from build123d import *

# Parameters (mm, degrees)
SCREW_HOLES_COUNT = 12


with BuildPart() as part:
    # Cross Section → Main (revolve)
    with BuildSketch(Plane.XY):
        Polygon((-38.1, 0), (-38.1, -3.175), (-41.275, -3.175), (-41.275, -15.875), (-41.656, -15.215088642), (-41.656, -3.175), (-48.514, -3.175), (-48.514, 9.525), (-47.625, 9.525), (-47.625, 0), align=None)
    revolve(axis=Axis((0, 55, 0), (0, -1, 0)))

    # Sketch7 → #3-48 Tapped Hole1 (revolve, cut)
    with BuildSketch(Plane(origin=(-42.8625, 0, 0), x_dir=(0, 0, 1), z_dir=(1, 0, 0))):
        Polygon((0, 0), (0, 3.901027994), (0.99695, 3.302), (0.99695, 0), align=None)
    f_3_48_tapped_hole1 = revolve(axis=Axis((-42.8625, 6.35, 0), (0, -1, 0)), mode=Mode.SUBTRACT)

    # Screw Holes: #3-48 Tapped Hole1 ×12 about axis
    screw_holes_axis = Axis((0, 0, 0), (0, 1, 0))
    for i in range(1, SCREW_HOLES_COUNT):
        add(f_3_48_tapped_hole1.rotate(screw_holes_axis, i * 360 / SCREW_HOLES_COUNT), mode=Mode.SUBTRACT)


solid = part.part
Source: CAD feature listing. Evaluate the final solid. Frame: model axes, mm. A direction names the side the tool comes from. Give positions to 0.01 mm unless a question says otherwise; leave off trailing zeros. Write each loop counter-clockwise with the first axis right and the second up, starting at its lowest first coordinate (ties: lowest second). Pieces come first, ordered by that corner, then holes. Notation, with made-up numbers: (49, 61) - (62, 61) arc R21 ccw to (62, 81) - close; hole circle Ø2 at (84.25, 6.25). An arc over 180 degrees is marked (long way). Write item = value, one per line. Start each with the question number.
Q1. Draft query along Z for faces 1 (the cylindrical face through (-46.274, 3.264, -14.572)), 2 (the cylindrical face through (30.235, -1.61, 23.183)), 3 (the flat face through (14, -3.175, -40)). Return one class per face: +Z half, -Z half, draft (parallel to the pull), parting line (faces both ways), or undercut.
Q2. Cut plane A-A, the plane y = -1.25. Give the number of separate pieces and of enclosed holes in the cut face, then the cut area to 3 significant figures.
Q3. Pin query (flat end, axial travel): pin 1 Ø2 at (x, y) = (23, -11) entering from -Z; pin 2 Ø1 at (y, z) = (6.5, -20.5) entering from -X; pin 3 Ø2.5 at (x, z) = (-37.12, 21.43) entering from +Y. Return the tip coordinate at first contact, or that it passes through.
Q4. Reachability of faces 4 (the flat face through (14, 0, -36)), 5 (the flat face through (-36, 9.525, 32)), 6 (the cylindrical face through (-39.732, -9.111, -12.512)) from +Z, -Z, +X, -X, +Y, -Y: full face, straight path, thin tool, end or side. Return the list, or none.
Q5. Material intervals for probe 1 along Z at (x, y) = (0, -1.7); probe 2 along X at (y, z) = (-2.75, -43); probe 3 along X at (y, z) = (-11.25, 1), sorted ascending.
Q6. Cut plane B-B, the plane y = -9.25. Return loops of the section in (x, z) (3 decimals).
Computed values:
q1.face_1 = parting line
q1.face_2 = undercut
q1.face_3 = draft
q2.separate_pieces = 1
q2.enclosed_holes = 13
q2.area = 2,800 mm²
q3.pin_1 = -35.37
q3.pin_2 = -44.2
q3.pin_3 = 0
q4.face_4 = +Y
q4.face_5 = +Z, -Z, +X, -X, +Y
q4.face_6 = -Y
q5.probe_1 = -48.51 to -43.86, -41.87 to -38.1, 38.1 to 41.87, 43.86 to 48.51
q5.probe_2 = -22.46 to -0.99, 0.99 to 22.46
q5.probe_3 = -41.64 to -41.26, 41.26 to 41.64
q6.outline = circle Ø83.312 at (0, 0); hole circle Ø82.55 at (0, 0)
